The drawing under review shows one solid part. Ordinate dimensions are in mm from its lowest x, y, z. Coordinates: 2 decimals unless noted, no trailing zeros. Order: outer loops, then holes, each group sorted by start corner. A loop starts at its lowest first (then second) coordinate and runs counter-clockwise, first axis right, second up. Notation, with made-up numbers: (-35.5, 33.5) - (-29.5, 33.5) arc R25 ccw to (-29.5, 72.5) - close; hole circle Ø2 at (-23, -12.75). An arc over 180 degrees is marked (long way). Write item = value, one per line. Start each with the question number.
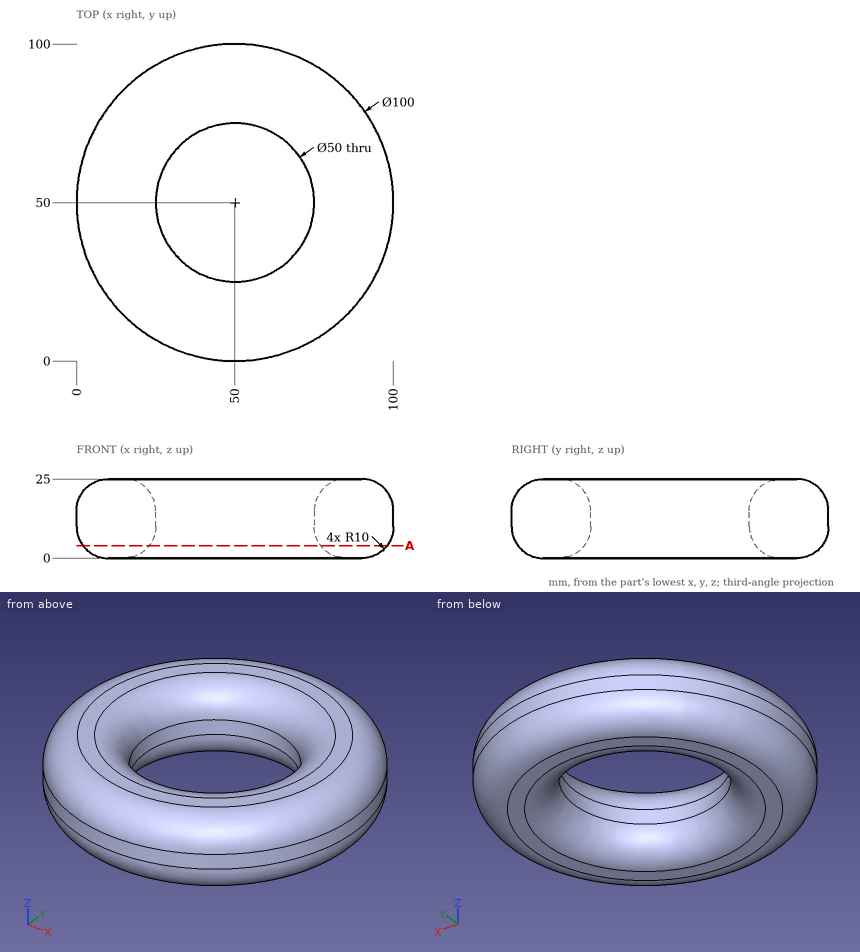
Item 1: For line 1 (Y direction, x = 50, z = 12.45); line 2 (Z direction, x = 24, y = 27); line 3 (Y direction, x = 29.5, z = 13.5), list the stretches that pass through material, from the lowest coordinate up.
Item 2: Add section A-A on z = 4. Give the boundary of the cut face in (x, y), plus the area to 3 significant figures.
Item 3: For P1, Ø6, axis at x = 17, z = 19, coming from the -Y side; P2, Ø4, axis at y = 58, z = 22, coming from the +X side; P3, Ø8, axis at x = 16.5, z = 21.5, coming from the +Y side; P4, Ø12, axis at y = 49.5, z = 4, coming from the +X side, all flat-tipped, find the tip position at first contact; note any pin that passes through.
Worked out:
q1.line_1 = 0 to 25, 75 to 100
q1.line_2 = 0 to 25
q1.line_3 = 4.4 to 35.69, 64.31 to 95.6
q2.outline = circle Ø96 at (50, 50); hole circle Ø54 at (50, 50)
q2.area = 4,950 mm2
q3.P1 = 10.69
q3.P2 = 98.04
q3.P3 = 88.66
q3.P4 = 100
